Part model, mm, in its own coordinate system. A direction names the side the tool comes from. Give positions to 0.01 mm unless a question says otherwise; leave off trailing zeros. Order: outer loops, then holes, each group sorted by start corner. A loop starts at its lowest first (then second) coordinate and runs counter-clockwise, first axis right, second up. Notation, with made-up numbers: M 13,-14 L 69,-14 A13 cw 69,6 Z; hole C -16,-16 d3. An arc over 180 degrees is marked long. One line per question, with ' | ' between items.
```python
from build123d import *

# Parameters (mm, degrees)
F1_DEPTH = 590.55
F3_DEPTH = 25.4


with BuildPart() as f1:
    # F0 (on Top) → F1 (new body)
    with BuildSketch(Plane.XY):
        with BuildLine():
            Line((100.850261, 44.084094), (100.850261, 50.434094))
            Line((100.850261, 50.434094), (-51.549739, 50.434094))
            Line((-51.549739, 50.434094), (-51.549739, -101.965906))
            Line((-51.549739, -101.965906), (-45.199739, -101.965906))
            ThreePointArc((-45.199739, -101.965906), (-40.709611, -100.106034), (-38.849739, -95.615906))
            Line((-38.849739, -95.615906), (-38.849739, 25.034094))
            ThreePointArc((-38.849739, 25.034094), (-35.129995, 34.01435), (-26.149739, 37.734094))
            Line((-26.149739, 37.734094), (94.500261, 37.734094))
            ThreePointArc((94.500261, 37.734094), (98.990389, 39.593966), (100.850261, 44.084094))
        make_face()
    extrude(amount=F1_DEPTH)

    # F2 (on face) → F3 (cut)
    with BuildSketch(Plane(origin=(0, 50.434094, 0), x_dir=(-1, 0, 0), z_dir=(0, 1, 0))):
        with BuildLine():
            ThreePointArc((-100.850261, 101.834363), (-26.195351, 186.025469), (0.749739, 295.275))
            ThreePointArc((0.749739, 295.275), (-26.195351, 404.524531), (-100.850261, 488.715637))
            Line((-100.850261, 488.715637), (-100.850261, 101.834363))
        make_face()
    extrude(amount=-F3_DEPTH, mode=Mode.SUBTRACT)


solid = f1.part
```
1. Tool access for faces 1 (the flat face through (-43, 8, 590.55)), 2 (the flat face through (-38.85, -36, 291)): list every direction of +Z, -Z, +X, -X, +Y, -Y with a clear straight run to the whole face (end or side of a thin tool).
Worked out:
face 1: +Z, +X, -X, +Y, -Y | face 2: +Z, -Z, +X, -Y
2. Slice it at C-C on y = -2. Give the cut face in (x, z), then the cut area to 3 significant figures.
Worked out:
outline: M -51.55,0 L -38.85,0 L -38.85,590.55 L -51.55,590.55 Z | area: 7,500 mm2
3. Slice it at D-D on z = 257. Give the cut face in (x, y), then the cut area to 3 significant figures.
Worked out:
outline: M -51.55,-101.97 L -45.2,-101.97 A6.35 ccw -38.85,-95.62 L -38.85,25.03 A12.7 cw -26.15,37.73 L 2.39,37.73 L 2.39,50.43 L -51.55,50.43 Z | area: 2,490 mm2
4. Slice it at A-A on x = 37. Give the cut face in (y, z).
Worked out:
outline: M 37.73,0 L 50.43,0 L 50.43,167.55 L 37.73,167.55 Z; M 37.73,423 L 50.43,423 L 50.43,590.55 L 37.73,590.55 Z
5. Probe L1, parallel to X at y = -59.5, z = 139; L2, parallel to Y at x = -23.5, z = 292. List the from-to ranges inside material, lowest first. Write a range as from..to.
Worked out:
L1: x = -51.55..-38.85 | L2: y = 37.73..50.43
6. Slice it at B-B on z = 475. Give the cut face in (x, y), then the cut area to 3 significant figures.
Worked out:
outline: M -51.55,-101.97 L -45.2,-101.97 A6.35 ccw -38.85,-95.62 L -38.85,25.03 A12.7 cw -26.15,37.73 L 82.87,37.73 L 82.87,50.43 L -51.55,50.43 Z | area: 3,510 mm2
7. Drop flat-ended pins along their axis: pin 1 (5 mm diameter, centred on y = -74, z = 324.5, fed in from +X); pin 2 (5 mm diameter, centred on x = 67, z = 466.5, fed in from -Y). Give the stop position or say it passes through.
Worked out:
pin 1: stops at x = -38.85 | pin 2: stops at y = 37.73
